Input: dimensioned drawing with shaded views. Units: mm. Origin: part minimum x, y, z. Round coordinates to 2 decimals unless told otherwise and drop trailing zeros. Loops run counter-clockwise (first coordinate to the right, second up) from the corner with the lowest first, then second, coordinate; pieces in that order, holes last. Notation, with made-up numbers: (82, -30) - (116, -30) arc R6 cw to (116, -19) - close; hole circle Ø10 at (48.5, -16.5). An arc over 180 degrees is marked (long way). One line per question, with ' | ' between items.
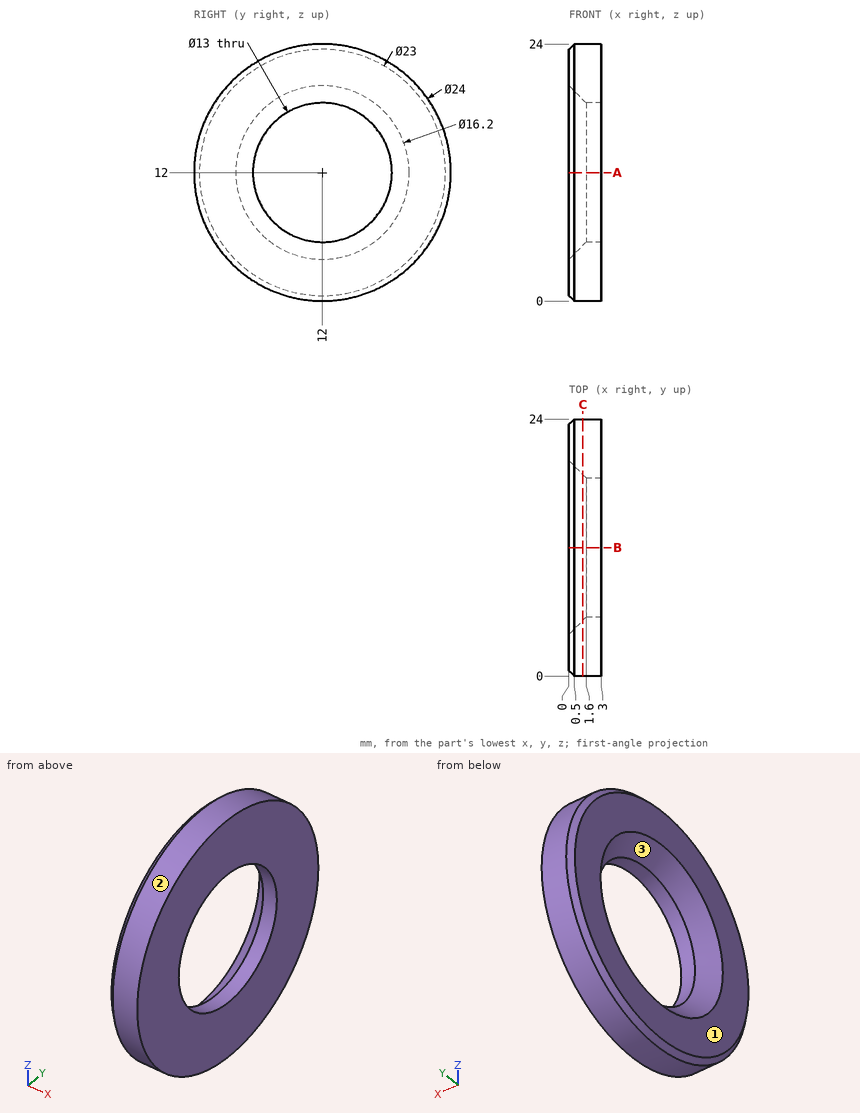
1. Section query C-C, the plane x = 1.3. Return loops of the section in (y, z), plus the area to 3 significant figures.
Worked out:
outline: circle Ø24 at (12, 12); hole circle Ø13.6 at (12, 12) | area: 307 mm2
2. Section query A-A, the plane z = 12. Return loops of the section in (x, y).
Worked out:
outline: (0, 0.5) - (0.5, 0) - (3, 0) - (3, 5.5) - (1.6, 5.5) - (0, 3.9) - close; (0, 20.1) - (1.6, 18.5) - (3, 18.5) - (3, 24) - (0.5, 24) - (0, 23.5) - close
3. Material intervals for probe 1 along Z at (x, y) = (2.6, 12); probe 2 along Z at (x, y) = (2.2, 15.75); probe 3 along Y at (x, z) = (2.55, 10), sorted ascending.
Worked out:
probe 1: z = 0 to 5.5, 18.5 to 24 | probe 2: z = 0.6 to 6.69, 17.31 to 23.4 | probe 3: y = 0.17 to 5.82, 18.18 to 23.83
4. Contact query for a flat-ended pin moving along its axis: P1, Ø8, axis at y = 12, z = 12, coming from the +X side. Output: stop coordinate, or through.
Worked out:
P1: passes through
5. Mould query, pull axis Z, two halves, no side actions, for the marked faces 1, 2 and 3. Classes: released by +Z, released by -Z, zero draft, split by the parting line, or undercut.
Worked out:
face 1: zero draft | face 2: split by the parting line | face 3: undercut
